For this review, take the finished solid that the model builds, in its own axes (mm). Face numbers are marked on the shaded views. Give positions to 0.01 mm unless a question says otherwise; leave off trailing zeros. Write each loop counter-clockwise with the first axis right and the second up, starting at its lowest first coordinate (ties: lowest second). Pieces come first, ordered by that corner, then holes. Notation, with made-up numbers: (37.5, 43.25) -> (96.5, 43.25) arc R20 ccw to (96.5, 53.25) -> close; hole circle Ø1 at (-2, -4). An arc over 180 degrees is marked (long way). Return JSON: item names as keys, results as strings.
Autodesk Inventor part; units mm, degrees
ref_plane "YZ Plane" through (0, 0, 0) normal (1, 0, 0) x (0, 1, 0)
ref_plane "XZ Plane" through (0, 0, 0) normal (0, 1, 0) x (-1, 0, 0)
ref_plane "XY Plane" through (0, 0, 0) normal (0, 0, 1) x (1, 0, 0)
sketch "Sketch1" plane through (0, 0, 0) normal (0, 1, 0) x (-1, 0, 0)
  line L0 (-50.8, -67.31) -> (50.8, -67.31)
  line L1 (50.8, -67.31) -> (50.8, 67.31)
  line L2 (50.8, 67.31) -> (-50.8, 67.31)
  line L3 (-50.8, 67.31) -> (-50.8, -67.31)
  line L4 (-50.8, -67.31) -> (50.8, 67.31) construction
  line L5 (50.8, -67.31) -> (-50.8, 67.31) construction
  point P0 (0, 0)
  dimension "d0" = 101.6
  dimension "d1" = 134.62
extrude "Extrusion1" add sketch "Sketch1" along normal blind 38.1
sketch "Sketch3" plane through (0, 38.1, 0) normal (0, 1, 0) x (1, 0, 0)
  line L0 (50.8, 63.5) -> (-50.8, 63.5)
  line L1 (-50.8, 63.5) -> (-50.8, -63.5)
  line L2 (-50.8, -63.5) -> (50.8, -63.5)
  line L3 (50.8, -63.5) -> (50.8, 63.5)
  line L4 (50.8, 63.5) -> (-50.8, -63.5) construction
  line L5 (-50.8, 63.5) -> (50.8, -63.5) construction
  point P0 (0, 0)
  dimension "d4" = 127
extrude "Extrusion2" cut sketch "Sketch3" against normal blind 34.29
sketch "Sketch4" plane through (50.8, 0, -67.31) normal (0, 0, -1) x (-1, 0, 0)
  line L0 (101.6, 38.1) -> (50.8, 38.1)
  line L1 (50.8, 38.1) -> (50.8, 0)
  line L2 (50.8, 0) -> (101.6, 0)
  line L3 (101.6, 0) -> (101.6, 38.1)
  dimension "d7" = 50.8
extrude "Extrusion3" cut sketch "Sketch4" against normal blind 5.08
sketch "Sketch5" plane through (-50.8, 0, 67.31) normal (0, 0, 1) x (1, 0, 0)
  line L0 (0, 38.1) -> (0, 3.81)
  line L1 (0, 38.1) -> (50.8, 38.1)
  line L2 (50.8, 38.1) -> (50.8, 0)
  line L3 (50.8, 0) -> (0, 0)
  line L4 (0, 0) -> (0, 38.1)
extrude "Extrusion4" cut sketch "Sketch5" against normal blind 5.08
sketch "Sketch6" plane through (50.8, 0, 67.31) normal (0, 0, 1) x (1, 0, 0)
  line L0 (-50.8, 38.1) -> (-38.1, 38.1)
  line L1 (-38.1, 38.1) -> (-38.1, 25.4)
  line L2 (-38.1, 25.4) -> (-50.8, 25.4)
  line L3 (-50.8, 25.4) -> (-50.8, 38.1)
  line L4 (0, 38.1) -> (-50.8, 38.1)
  line L5 (0, 38.1) -> (-12.7, 38.1)
  line L6 (-12.7, 38.1) -> (-12.7, 25.4)
  line L7 (-12.7, 25.4) -> (0, 25.4)
  line L8 (0, 25.4) -> (0, 38.1)
  point P0 (-50.8, 0)
  dimension "d12" = 12.7
  dimension "d13" = 12.7
  dimension "d14" = 12.7
hole "Hole1" at (12.7, 25.4, 67.31) at (38.1, 25.4, 67.31) direction (0, 0, -1) diameter 3.7 end through all
sketch "Sketch8" plane through (0, 0, 0) normal (0, -1, 0) x (1, 0, 0)
  circle A0 centre (-18.8, -24.23) radius 1.85
  circle A1 centre (-34.8, -24.23) radius 1.85
  circle A2 centre (-18.8, -40.23) radius 1.85
  circle A3 centre (-34.8, -40.23) radius 1.85
  point P0 (0, 0)
hole "Hole2" at (-18.8, 0, -24.23) at (-34.8, 0, -24.23) at (-34.8, 0, -40.23) at (-18.8, 0, -40.23) direction (0, 1, 0) diameter 3.7 end through all
properties part number "Bucket Top" material "PET Plastic"
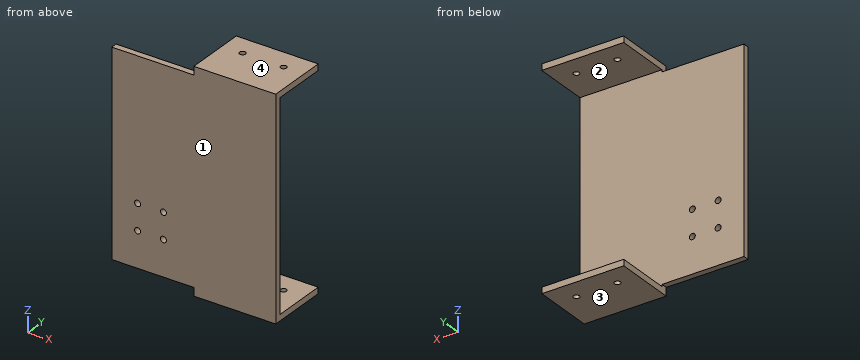
1. To check wall thickness, follow probe 1 along X at (y, z) = (25.4, 66.05); probe 2 along X at (y, z) = (2, -40); probe 3 along Z at (x, y) = (39, 19.5). State the ranges of each line that lie inside material, in increasing order.
Results found:
{"probe 1": "x = 0 to 10.85, 14.55 to 36.25, 39.95 to 50.8", "probe 2": "x = -50.8 to -36.64, -32.96 to -20.64, -16.96 to 50.8", "probe 3": "z = -67.31 to -63.5, 63.5 to 67.31"}
2. Add section A-A, the plane x = -34.8. State the section outline as (y, z) points.
Results found:
{"outline": "(0, -62.23) -> (3.81, -62.23) -> (3.81, -42.08) -> (0, -42.08) -> close; (0, -38.38) -> (3.81, -38.38) -> (3.81, -26.08) -> (0, -26.08) -> close; (0, -22.38) -> (3.81, -22.38) -> (3.81, 62.23) -> (0, 62.23) -> close"}
3. Add section B-B, the plane z = -40.23. State the section outline as (x, y) points, plus the area to 3 significant figures.
Results found:
{"outline": "(-50.8, 0) -> (-36.65, 0) -> (-36.65, 3.81) -> (-50.8, 3.81) -> close; (-32.95, 0) -> (-20.65, 0) -> (-20.65, 3.81) -> (-32.95, 3.81) -> close; (-16.95, 0) -> (50.8, 0) -> (50.8, 3.81) -> (-16.95, 3.81) -> close", "area": "359 mm²"}
4. Add section D-D, the plane y = 25.4. State the section outline as (x, z) points.
Results found:
{"outline": "(0, -67.31) -> (10.85, -67.31) -> (10.85, -63.5) -> (0, -63.5) -> close; (0, 63.5) -> (10.85, 63.5) -> (10.85, 67.31) -> (0, 67.31) -> close; (14.55, -67.31) -> (36.25, -67.31) -> (36.25, -63.5) -> (14.55, -63.5) -> close; (14.55, 63.5) -> (36.25, 63.5) -> (36.25, 67.31) -> (14.55, 67.31) -> close; (39.95, -67.31) -> (50.8, -67.31) -> (50.8, -63.5) -> (39.95, -63.5) -> close; (39.95, 63.5) -> (50.8, 63.5) -> (50.8, 67.31) -> (39.95, 67.31) -> close"}
5. Add section C-C, the plane y = 33.5. State the section outline as (x, z) points.
Results found:
{"outline": "(0, -67.31) -> (50.8, -67.31) -> (50.8, -63.5) -> (0, -63.5) -> close; (0, 63.5) -> (50.8, 63.5) -> (50.8, 67.31) -> (0, 67.31) -> close"}
6. For pin 1 (1.1 mm diameter, centred on x = -32.5, y = 2, fed in from +Z); pin 2 (3 mm diameter, centred on x = -31.5, z = -43, fed in from +Y); pin 3 (4 mm diameter, centred on y = 17, z = -64, fed in from -X), all flat-tipped, find the tip position at first contact; note any pin that passes through.
Results found:
{"pin 1": "stops at z = 62.23", "pin 2": "stops at y = 3.81", "pin 3": "stops at x = 0"}
7. The part is to be moulded in two halves that separate along Z. For the marked faces 1, 2, 3 and 4, say which applies: +Z half, -Z half, draft (parallel to the pull), parting line (faces both ways), or undercut.
Results found:
{"face 1": "draft", "face 2": "undercut", "face 3": "-Z half", "face 4": "+Z half"}
